from build123d import *

# Parameters (mm, degrees)
SKETCH1_W           = 80
SKETCH1_H           = 36
BOSS_EXTRUDE1_DEPTH = 1.6
SKETCH2_W           = 71.2
SKETCH2_H           = 25.2
BOSS_EXTRUDE2_DEPTH = 8.6
SKETCH3_R           = 1.5
CUT_EXTRUDE3_DEPTH  = 13.2
SKETCH6_W           = 66
SKETCH6_H           = 16
CUT_EXTRUDE4_DEPTH  = 1
SKETCH7_R           = 0.5
CUT_EXTRUDE5_DEPTH  = 21


with BuildPart() as part:
    # Sketch1 → Boss-Extrude1 (new body)
    with BuildSketch(Plane(origin=(0, 0, 0), x_dir=(1, 0, 0), z_dir=(0, 1, 0))):
        with Locations((3.287671233, 10.219178082)):
            Rectangle(SKETCH1_W, SKETCH1_H)
    extrude(amount=BOSS_EXTRUDE1_DEPTH)

    # Sketch2 → Boss-Extrude2 (add)
    with BuildSketch(Plane(origin=(0, 1.6, 0), x_dir=(1, 0, 0), z_dir=(0, 1, 0))):
        with Locations((3.837671233, 10.419178082)):
            Rectangle(SKETCH2_W, SKETCH2_H)
    extrude(amount=BOSS_EXTRUDE2_DEPTH)

    # Sketch3 → Cut-Extrude3 (cut)
    with BuildSketch(Plane(origin=(0, 1.6, 0), x_dir=(1, 0, 0), z_dir=(0, 1, 0))):
        with Locations(Location((-33.712328767, 25.719178082, 0), (0, 0, 270))):
            Circle(SKETCH3_R)
        with Locations(Location((41.287671233, 25.719178082, 0), (0, 0, 270))):
            Circle(SKETCH3_R)
        with Locations(Location((-33.712328767, -5.280821918, 0), (0, 0, 270))):
            Circle(SKETCH3_R)
        with Locations(Location((41.287671233, -5.280821918, 0), (0, 0, 270))):
            Circle(SKETCH3_R)
    extrude(amount=-CUT_EXTRUDE3_DEPTH, mode=Mode.SUBTRACT)

    # Sketch6 → Cut-Extrude4 (cut)
    with BuildSketch(Plane(origin=(0, 10.2, 0), x_dir=(1, 0, 0), z_dir=(0, 1, 0))):
        with Locations((4.287671233, 10.419178082)):
            Rectangle(SKETCH6_W, SKETCH6_H)
    extrude(amount=-CUT_EXTRUDE4_DEPTH, mode=Mode.SUBTRACT)

    # Sketch7 → Cut-Extrude5 (cut)
    with BuildSketch(Plane(origin=(0, 1.6, 0), x_dir=(1, 0, 0), z_dir=(0, 1, 0))):
        with Locations(Location((-28.712328767, 25.719178082, 0), (0, 0, 270))):
            Circle(SKETCH7_R)
        with Locations(Location((-26.172328767, 25.719178082, 0), (0, 0, 270))):
            Circle(SKETCH7_R)
        with Locations(Location((-23.632328767, 25.719178082, 0), (0, 0, 270))):
            Circle(SKETCH7_R)
        with Locations(Location((-21.092328767, 25.719178082, 0), (0, 0, 270))):
            Circle(SKETCH7_R)
        with Locations(Location((-18.552328767, 25.719178082, 0), (0, 0, 270))):
            Circle(SKETCH7_R)
        with Locations(Location((-16.012328767, 25.719178082, 0), (0, 0, 270))):
            Circle(SKETCH7_R)
        with Locations(Location((-13.472328767, 25.719178082, 0), (0, 0, 270))):
            Circle(SKETCH7_R)
        with Locations(Location((-10.932328767, 25.719178082, 0), (0, 0, 270))):
            Circle(SKETCH7_R)
        with Locations(Location((-8.392328767, 25.719178082, 0), (0, 0, 270))):
            Circle(SKETCH7_R)
        with Locations(Location((-5.852328767, 25.719178082, 0), (0, 0, 270))):
            Circle(SKETCH7_R)
        with Locations(Location((-3.312328767, 25.719178082, 0), (0, 0, 270))):
            Circle(SKETCH7_R)
        with Locations(Location((-0.772328767, 25.719178082, 0), (0, 0, 270))):
            Circle(SKETCH7_R)
        with Locations(Location((1.767671233, 25.719178082, 0), (0, 0, 270))):
            Circle(SKETCH7_R)
        with Locations(Location((4.307671233, 25.719178082, 0), (0, 0, 270))):
            Circle(SKETCH7_R)
        with Locations(Location((6.847671233, 25.719178082, 0), (0, 0, 270))):
            Circle(SKETCH7_R)
        with Locations(Location((9.387671233, 25.719178082, 0), (0, 0, 270))):
            Circle(SKETCH7_R)
    extrude(amount=-CUT_EXTRUDE5_DEPTH, mode=Mode.SUBTRACT)


solid = part.part
Input: part model. Units: mm. Frame: model coordinates. A direction names the side the tool comes from. Coordinates: 2 decimals unless noted, no trailing zeros. Order: outer loops, then holes, each group sorted by start corner. A loop starts at its lowest first (then second) coordinate and runs counter-clockwise, first axis right, second up.
1. Cut plane B-B, the plane x = 36.5. Return loops of the section in (y, z).
Checked values:
outline: (0, -28.22) - (1.6, -28.22) - (1.6, -23.02) - (10.2, -23.02) - (10.2, -18.42) - (9.2, -18.42) - (9.2, -2.42) - (10.2, -2.42) - (10.2, 2.18) - (1.6, 2.18) - (1.6, 7.78) - (0, 7.78) - close
2. Draft query along X for faces 1 (the cylindrical face through (-35.177, 0.811, 4.956)), 2 (the flat face through (43.288, 1, -10)), 3 (the flat face through (3, 1, -28.219)). Return one class per face: +X half, -X half, draft (parallel to the pull), parting line (faces both ways), or undercut.
Checked values:
face 1: undercut
face 2: +X half
face 3: draft
3. Access query for faces 4 (the flat face through (4, 9.2, -11)), 5 (the flat face through (3, 6, 2.181)), 6 (the flat face through (-31.762, 6, -10)), 7 (the flat face through (3, 6, -23.019)). Directions: +Z, -Z, +X, -X, +Y, -Y. A direction counts if a zero-diameter tool reaches every point of the face in a straight line with its end or side. Return the directions, or none.
Checked values:
face 4: +Y
face 5: +Z, +X, -X, +Y
face 6: +Z, -Z, -X, +Y
face 7: -Z, +X, -X, +Y
4. Contact query for flat-ended pins moving along their axis: P1, Ø2, axis at x = 18, y = 8, coming from the -Z side; P2, Ø1.5, axis at x = 12.5, z = -11.5, coming from the +Y side; P3, Ø0.8, axis at y = 9.5, z = -8, coming from the +X side. Output: stop coordinate, or through.
Checked values:
P1: stops at z = -23.02
P2: stops at y = 9.2
P3: stops at x = 39.44
5. Cut plane D-D, the plane y = 5.5. Return loops of the section in (x, z).
Checked values:
outline: (-31.76, -23.02) - (39.44, -23.02) - (39.44, 2.18) - (-31.76, 2.18) - close
6. Cut plane C-C, the plane z = 5. Return loops of the section in (x, y), plus the area to 3 significant figures.
Checked values:
outline: (-36.71, 0) - (-35.19, 0) - (-35.19, 1.6) - (-36.71, 1.6) - close; (-32.24, 0) - (39.81, 0) - (39.81, 1.6) - (-32.24, 1.6) - close; (42.76, 0) - (43.29, 0) - (43.29, 1.6) - (42.76, 1.6) - close
area: 119 mm2
7. Ray query, line 1 along X through (y, z) = (0.5, 4); line 2 along Z through (x, y) = (37.5, 9.5); line 3 along X through (y, z) = (7.25, 1.5). Return the intervals inside material, ascending.
Checked values:
line 1: x = -36.71 to -34.49, -32.93 to 40.51, 42.07 to 43.29
line 2: z = -23.02 to 2.18
line 3: x = -31.76 to 39.44
8. Cut plane A-A, the plane z = -14.5. Return loops of the section in (x, y).
Checked values:
outline: (-36.71, 0) - (43.29, 0) - (43.29, 1.6) - (39.44, 1.6) - (39.44, 10.2) - (37.29, 10.2) - (37.29, 9.2) - (-28.71, 9.2) - (-28.71, 10.2) - (-31.76, 10.2) - (-31.76, 1.6) - (-36.71, 1.6) - close
